Geometry check sheet. Reference: the model listing, model coordinates, mm. A direction names the side the tool comes from. Round coordinates to 2 decimals unless told otherwise and drop trailing zeros. Write each loop counter-clockwise with the first axis right and the second up, starting at its lowest first coordinate (ties: lowest second). Pieces come first, ordered by that corner, then holes. Notation, with made-up numbers: M 31,85 L 65,85 A27 cw 65,111 Z; hole C 45,-31.5 d8. An arc over 180 degrees is marked long. Put each result on its own line as item: value. Start each with the question number.
(1) Tool access check on faces 1 (the flat face through (-5.85, 16, 5)), 2 (the flat face through (5, 10.8, 4.1)), 3 (the flat face through (6, 10.75, 3)), 4 (the flat face through (-2.7, 1, 4)). Record the directions out of +Z, -Z, +X, -X, +Y, -Y that give a thin tool (end or side, any length) a straight path to the whole face; none if there is none.
(2) Section check B-B on x = 0.5. Record the cut outline in (y, z).
(3) Mould release check, pull along Y, two halves, no side actions. Record for faces 5 (the flat face through (-5, 10, 3)), 6 (the cylindrical face through (5.5, 5.07, 0.79)), 7 (the flat face through (-3.85, 10.5, 3.8)): pulls with the +Y half, pulls with the -Y half, needs draft (parallel to the pull), parting line crosses it, or undercut.
(4) Section check D-D on x = 4. Record the cut outline in (y, z).
(5) Section check A-A on z = 3.5. Record the cut outline in (x, y) (3 decimals).
(6) Gauge pin test, flat ends, axial feed: pin 1 (1 mm diameter, centred on x = -5, z = 2.5, fed in from +Y); pin 2 (3 mm diameter, centred on y = 3, z = 5, fed in from -X); pin 3 (1.8 mm diameter, centred on y = 17, z = 5, fed in from -X); pin 4 (1.5 mm diameter, centred on y = 12, z = 3, fed in from +X). Record the tip position at first contact, or that the pin passes through.
(7) Material ranges on probe 1 along Y at (x, z) = (7, 0.6); probe 2 along Y at (x, z) = (-4.75, 2); probe 3 along Z at (x, y) = (-5, 8.5), recorded low to high.
(8) Section check C-C on y = 14. Record the cut outline in (x, z).
from build123d import *

# Parameters (mm, degrees)
SKETCH1_R           = 1.5
BOSS_EXTRUDE1_DEPTH = 1.6
SKETCH2_W           = 12.85
SKETCH2_H           = 10
BOSS_EXTRUDE2_DEPTH = 6
SKETCH3_W           = 12.85
SKETCH3_H           = 3
CUT_EXTRUDE1_DEPTH  = 3
CUT_EXTRUDE3_DEPTH  = 3
SKETCH5_W           = 2.25
SKETCH5_H           = 2.25
CUT_EXTRUDE4_DEPTH  = 17
BOSS_EXTRUDE4_DEPTH = 4.75
SKETCH11_W          = 12.85
SKETCH11_H          = 1.15
CUT_EXTRUDE8_DEPTH  = 4.75
SKETCH_1_W          = 5.7
SKETCH_1_H          = 7
EXTRUDE_1_DEPTH     = 5.8


with BuildPart() as part:
    # Sketch1 → Boss-Extrude1 (new body)
    with BuildSketch(Plane.XY):
        with BuildLine():
            Line((-7, 20), (7, 20))
            ThreePointArc((7, 20), (8.414213562, 19.414213562), (9, 18))
            Line((9, 18), (9, 2))
            ThreePointArc((9, 2), (8.414213562, 0.585786438), (7, 0))
            Line((7, 0), (-7, 0))
            ThreePointArc((-7, 0), (-8.414213562, 0.585786438), (-9, 2))
            Line((-9, 2), (-9, 18))
            ThreePointArc((-9, 18), (-8.414213562, 19.414213562), (-7, 20))
        make_face()
        with Locations((7, 5)):
            Circle(SKETCH1_R, mode=Mode.SUBTRACT)
        with Locations((-7, 5)):
            Circle(SKETCH1_R, mode=Mode.SUBTRACT)
    extrude(amount=BOSS_EXTRUDE1_DEPTH)

    # Sketch2 → Boss-Extrude2 (add)
    with BuildSketch(Plane.XY.offset(1.6)):
        with Locations((0.575, 15)):
            Rectangle(SKETCH2_W, SKETCH2_H)
    extrude(amount=BOSS_EXTRUDE2_DEPTH)

    # Sketch3 → Cut-Extrude1 (cut)
    with BuildSketch(Plane.XY.offset(7.6)):
        with Locations((0.575, 11.5)):
            Rectangle(SKETCH3_W, SKETCH3_H)
    extrude(amount=-CUT_EXTRUDE1_DEPTH, mode=Mode.SUBTRACT)

    # Sketch4 → Cut-Extrude3 (cut)
    with BuildSketch(Plane.XY.offset(4.6)):
        Polygon((5, 13), (1.575, 13), (1.575, 10), (5, 10), (5, 11.5), align=None)
        Polygon((-0.425, 13), (-3.85, 13), (-3.85, 11.5), (-3.85, 10), (-0.425, 10), align=None)
    extrude(amount=-CUT_EXTRUDE3_DEPTH, mode=Mode.SUBTRACT)

    # Sketch5 → Cut-Extrude4 (cut, through all)
    with BuildSketch(Plane(origin=(7, 0, 0), x_dir=(0, 0, -1), z_dir=(1, 0, 0))):
        with Locations((-2.725, 11.875)):
            Rectangle(SKETCH5_W, SKETCH5_H)
    extrude(amount=-CUT_EXTRUDE4_DEPTH, mode=Mode.SUBTRACT)

    # Sketch10 → Boss-Extrude4 (add)
    with BuildSketch(Plane.XY.offset(7.6)):
        Polygon((6.995, 23.262214419), (-5.85, 20), (-5.45, 20), (6.995, 23.16062736), align=None)
    extrude(amount=-BOSS_EXTRUDE4_DEPTH)

    # Sketch11 → Cut-Extrude8 (cut)
    with BuildSketch(Plane(origin=(0, 20, 0), x_dir=(1, 0, 0), z_dir=(0, 1, 0))):
        with Locations((0.575, -7.025)):
            Rectangle(SKETCH11_W, SKETCH11_H)
    extrude(amount=CUT_EXTRUDE8_DEPTH, mode=Mode.SUBTRACT)

    # 草图1 → 凸台-拉伸1 (add)
    with BuildSketch(Plane.XY.offset(1.6)):
        with Locations((0.15, 1.5)):
            Rectangle(SKETCH_1_W, SKETCH_1_H)
    extrude(amount=EXTRUDE_1_DEPTH)


solid = part.part
Answers follow:
1. face 1: +Z, -X, +Y, -Y
1. face 2: +Z, -Y
1. face 3: +X, -X
1. face 4: +Z, -X, -Y
2. outline: M -2,1.6 L 0,1.6 L 0,0 L 20,0 L 20,7.6 L 13,7.6 L 13,4.6 L 10,4.6 L 10,1.6 L 5,1.6 L 5,7.4 L -2,7.4 Z; M 21.51,2.85 L 21.61,2.85 L 21.61,6.45 L 21.51,6.45 Z; hole M 10.75,1.6 L 13,1.6 L 13,3.85 L 10.75,3.85 Z
3. face 5: pulls with the -Y half
3. face 6: undercut
3. face 7: needs draft
4. outline: M 0,0 L 20,0 L 20,7.6 L 13,7.6 L 13,1.6 L 0,1.6 Z; M 22.4,2.85 L 22.5,2.85 L 22.5,6.45 L 22.4,6.45 Z
5. outline: M -5.85,10 L -3.85,10 L -3.85,10.75 L -5.85,10.75 Z; M -5.85,13 L 7,13 L 7,20 L -5.45,20 L 6.995,23.161 L 6.995,23.262 L -5.85,20 Z; M -2.7,-2 L 3,-2 L 3,5 L -2.7,5 Z; M -0.425,10 L 1.575,10 L 1.575,10.75 L -0.425,10.75 Z; M 5,10 L 7,10 L 7,10.75 L 5,10.75 Z
6. pin 1: stops at y = 20.31
6. pin 2: stops at x = -2.7
6. pin 3: stops at x = -5.85
6. pin 4: passes through
7. probe 1: y = 0 to 3.5, 6.5 to 20
7. probe 2: y = 10 to 10.75, 13 to 20
7. probe 3: z = 0 to 1.6
8. outline: M -9,0 L 9,0 L 9,1.6 L 7,1.6 L 7,7.6 L -5.85,7.6 L -5.85,1.6 L -9,1.6 Z
